CAD build for the part. Positions are in the model's coordinates, mm. A direction names the side the tool comes from. Coordinates: 2 decimals unless noted, no trailing zeros. Order: outer loops, then holes, each group sorted by start corner. A loop starts at its lowest first (then second) coordinate and runs counter-clockwise, first axis right, second up. Notation, with made-up numbers: (16, 20.25) - (70, 20.25) arc R21 ccw to (70, 58.25) - close; hole circle Ø11 at (24, -1). An arc over 180 degrees is marked (long way). Use one line per item in the form item = value.
```python
from build123d import *

# Parameters (mm, degrees)
SKETCH1_W                = 90
SKETCH1_H                = 8.5
BOSS_EXTRUDE1_DEPTH      = 8.5
SKETCH2_W                = 8.5
SKETCH2_H                = 8.5
BOSS_EXTRUDE2_DEPTH      = 25.4
BOSS_EXTRUDE2_DEPTH_BACK = 33.9
SKETCH3_W                = 10.25
SKETCH3_H                = 8.5
BOSS_EXTRUDE3_DEPTH      = 25.4
BOSS_EXTRUDE3_DEPTH_BACK = 37.900000018
SKETCH4_W                = 8.5
SKETCH4_H                = 4
BOSS_EXTRUDE4_DEPTH      = 12.7
SKETCH5_W                = 8.5
SKETCH5_H                = 4
BOSS_EXTRUDE5_DEPTH      = 12.7
SKETCH6_R                = 2.032
CUT_EXTRUDE1_DEPTH       = 12.7
CUT_EXTRUDE2_DEPTH       = 9.906
CUT_EXTRUDE2_DEPTH_BACK  = 73.406
FILLET2_R                = 1.651


with BuildPart() as part:
    # Sketch1 → Boss-Extrude1 (new body)
    with BuildSketch(Plane.XY):
        Rectangle(SKETCH1_W, SKETCH1_H)
    extrude(amount=BOSS_EXTRUDE1_DEPTH)

    # Sketch2 → Boss-Extrude2 (add, two sides)
    with BuildSketch(Plane(origin=(0, 4.25, 0), x_dir=(1, 0, 0), z_dir=(0, 1, 0))) as boss_extrude2_sk:
        with Locations((13, -4.25)):
            Rectangle(SKETCH2_W, SKETCH2_H)
        with Locations((-13, -4.25)):
            Rectangle(SKETCH2_W, SKETCH2_H)
    extrude(amount=BOSS_EXTRUDE2_DEPTH)
    extrude(boss_extrude2_sk.sketch, amount=-BOSS_EXTRUDE2_DEPTH_BACK)

    # Sketch3 → Boss-Extrude3 (add, two sides)
    with BuildSketch(Plane(origin=(0, 4.25, 0), x_dir=(1, 0, 0), z_dir=(0, 1, 0))) as boss_extrude3_sk:
        with Locations((-39.875, -4.25)):
            Rectangle(SKETCH3_W, SKETCH3_H)
        with Locations((39.875, -4.25)):
            Rectangle(SKETCH3_W, SKETCH3_H)
    extrude(amount=BOSS_EXTRUDE3_DEPTH)
    extrude(boss_extrude3_sk.sketch, amount=-BOSS_EXTRUDE3_DEPTH_BACK)

    # Sketch4 → Boss-Extrude4 (add)
    with BuildSketch(Plane(origin=(45, 0, 0), x_dir=(0, 0, -1), z_dir=(1, 0, 0))):
        with Locations((-4.25, -31.650000018)):
            Rectangle(SKETCH4_W, SKETCH4_H)
    extrude(amount=BOSS_EXTRUDE4_DEPTH)

    # Sketch5 → Boss-Extrude5 (add)
    with BuildSketch(Plane.ZY.offset(45)):
        with Locations((4.25, -31.650000018)):
            Rectangle(SKETCH5_W, SKETCH5_H)
    extrude(amount=BOSS_EXTRUDE5_DEPTH)

    # Sketch6 → Cut-Extrude1 (cut)
    with BuildSketch(Plane(origin=(0, -29.650000018, 0), x_dir=(1, 0, 0), z_dir=(0, 1, 0))):
        with Locations((51.35, -4.25)):
            Circle(SKETCH6_R)
        with Locations((-51.35, -4.25)):
            Circle(SKETCH6_R)
    extrude(amount=-CUT_EXTRUDE1_DEPTH, mode=Mode.SUBTRACT)

    # Sketch7 → Cut-Extrude2 (cut, two sides)
    with BuildSketch(Plane(origin=(0, 29.65, 0), x_dir=(1, 0, 0), z_dir=(0, 1, 0))) as cut_extrude2_sk:
        Polygon((14.27, 0), (14.27, -1.27), (15.54, -1.27), (15.54, -3.175), (10.46, -3.175), (10.46, -1.27), (11.73, -1.27), (11.73, 0), align=None)
        Polygon((-11.73, -1.27), (-11.73, 0), (-14.27, 0), (-14.27, -1.27), (-15.54, -1.27), (-15.54, -3.175), (-10.46, -3.175), (-10.46, -1.27), align=None)
        Polygon((-14.27, -8.5), (-14.27, -7.23), (-15.54, -7.23), (-15.54, -5.325), (-10.46, -5.325), (-10.46, -7.23), (-11.73, -7.23), (-11.73, -8.5), align=None)
        Polygon((11.73, -7.23), (11.73, -8.5), (14.27, -8.5), (14.27, -7.23), (15.54, -7.23), (15.54, -5.325), (10.46, -5.325), (10.46, -7.23), align=None)
    extrude(amount=CUT_EXTRUDE2_DEPTH, mode=Mode.SUBTRACT)
    extrude(cut_extrude2_sk.sketch, amount=-CUT_EXTRUDE2_DEPTH_BACK, mode=Mode.SUBTRACT)

    # Fillet2
    fillet2_edges = [part.edges().sort_by_distance(p)[0] for p in [
        (57.7, -31.650000018, 8.5),
        (57.7, -33.650000018, 4.25),
        (57.7, -31.650000018, 0),
        (57.7, -29.650000018, 4.25),
        (-57.7, -31.650000018, 8.5),
        (-57.7, -29.650000018, 4.25),
        (-57.7, -31.650000018, 0),
        (-57.7, -33.650000018, 4.25),
        (26, -4.25, 0),
        (0, 4.25, 0),
        (0, 4.25, 8.5),
        (26, -4.25, 8.5),
        (0, -4.25, 0),
        (-26, 4.25, 0),
        (-26, 4.25, 8.5),
        (0, -4.25, 8.5),
        (-26, -4.25, 0),
        (-26, -4.25, 8.5),
        (-34.75, 16.95, 8.5),
        (-34.75, -18.950000009, 8.5),
        (-34.75, 16.95, 0),
        (-34.75, -18.950000009, 0),
        (-39.875, 29.65, 0),
        (-45, 29.65, 4.25),
        (-39.875, 29.65, 8.5),
        (-34.75, 29.65, 4.25),
        (26, 4.25, 0),
        (26, 4.25, 8.5),
        (34.75, 16.95, 0),
        (34.75, -18.950000009, 0),
        (34.75, 16.95, 8.5),
        (34.75, -18.950000009, 8.5),
        (39.875, 29.65, 0),
        (34.75, 29.65, 4.25),
        (39.875, 29.65, 8.5),
        (45, 29.65, 4.25),
    ]]
    fillet(fillet2_edges, radius=FILLET2_R)


solid = part.part
```
Item 1: Drill centre lines: line 1 (X direction, y = 18.5, z = 6.5); line 2 (X direction, y = -3, z = 0.5); line 3 (X direction, y = 3.5, z = 3). Where is each one in solid material? Low to high. Write a range as [from, to].
Derived:
line_1 = [-45, -34.75], [-17.25, -15.54], [-10.46, -8.75], [8.75, 10.46], [15.54, 17.25], [34.75, 45]
line_2 = [-45, -14.27], [-11.73, 11.73], [14.27, 45]
line_3 = [-45, -15.54], [-10.46, 10.46], [15.54, 45]
Item 2: Cut at C-C, the plane x = -32. Write the cut outline in (y, z).
Derived:
outline = (-4.25, 1.65) arc R1.65 ccw to (-2.6, 0) - (2.6, 0) arc R1.65 ccw to (4.25, 1.65) - (4.25, 6.85) arc R1.65 ccw to (2.6, 8.5) - (-2.6, 8.5) arc R1.65 ccw to (-4.25, 6.85) - close
Item 3: Drop flat-ended pins along their axis: pin 1 (1.6 mm diameter, centred on y = -18, z = 4, fed in from +X); pin 2 (2 mm diameter, centred on y = 9, z = 6.5, fed in from -X); pin 3 (3 mm diameter, centred on x = -31, z = 6, fed in from -Y). Give the stop position or say it passes through.
Derived:
pin_1 = 45
pin_2 = -45
pin_3 = -4.25
Item 4: 3-axis set-ups, long thin cutter, end or side, ignore diameter. For faces 1 (the face through (-26, -4.25, 4)), 2 (the face through (-49, -29.65, 4)), 3 (the face through (0, 4.25, 4)): which of +Z, -Z, +X, -X, +Y, -Y reach the whole face in a straight line?
Derived:
face_1 = +Z, -Z, -Y
face_2 = +Z, -Z, -X, +Y
face_3 = +Z, -Z, +Y
Item 5: Two-plate mould, pull along Z, no slides. Class faces 4 (the face through (49.32, -31.62, 4.16)), 5 (the face through (-35, -2, 0)), 6 (the face through (-45, -33.65, 4)): +Z half, -Z half, draft (parallel to the pull), parting line (faces both ways), or undercut.
Derived:
face_4 = undercut
face_5 = -Z half
face_6 = draft
Item 6: Cut at A-A, the plane x = -51.35. Write the cut outline in (y, z), plus the area to 3 significant figures.
Derived:
outline = (-33.65, 0) - (-29.65, 0) - (-29.65, 2.22) - (-33.65, 2.22) - close; (-33.65, 6.28) - (-29.65, 6.28) - (-29.65, 8.5) - (-33.65, 8.5) - close
area = 17.7 mm²
Item 7: Cut at B-B, the plane y = 14. State how many separate pieces and enclosed holes the cut face has, plus the area to 3 significant figures.
Derived:
separate_pieces = 4
enclosed_holes = 0
area = 265 mm²
